Check sheet for the modelled part. Datum: model origin and axes. Units: mm. A direction names the side the tool comes from. Round coordinates to 2 decimals unless told otherwise and drop trailing zeros. Order: outer loops, then holes, each group sorted by start corner. A loop starts at its lowest first (then second) coordinate and runs counter-clockwise, first axis right, second up.
```python
from build123d import *

# Parameters (mm, degrees)
SKETCH_W     = 34
SKETCH_H     = 20
PAD_DEPTH    = 15
SKETCH001_R  = 0.8
PAD001_DEPTH = 2
FILLET_R     = 1
FILLET001_R  = 0.5


with BuildPart() as part:
    # Sketch → Pad (new body)
    with BuildSketch(Plane.XZ):
        with Locations((18.71189, -10.724301)):
            Rectangle(SKETCH_W, SKETCH_H)
    extrude(amount=PAD_DEPTH)

    # Sketch001 → Pad001 (join)
    with BuildSketch(Plane.XZ):
        with Locations((4.01189, -13.224301)):
            Circle(SKETCH001_R)
        with Locations((4.01189, -8.224301)):
            Circle(SKETCH001_R)
        with Locations((33.41189, -18.424301)):
            Circle(SKETCH001_R)
        with Locations((33.41189, -3.024301)):
            Circle(SKETCH001_R)
    extrude(amount=-PAD001_DEPTH)

    # Fillet
    fillet_edges = [part.edges().sort_by_distance(p)[0] for p in [
        (35.71189, -7.5, -20.724301),
        (18.71189, -15, -20.724301),
        (1.71189, -7.5, -20.724301),
        (18.71189, 0, -20.724301),
        (35.71189, -15, -10.724301),
        (35.71189, 0, -10.724301),
        (18.71189, -15, -0.724301),
        (35.71189, -7.5, -0.724301),
        (1.71189, -7.5, -0.724301),
        (1.71189, -15, -10.724301),
        (1.71189, 0, -10.724301),
        (18.71189, 0, -0.724301),
    ]]
    fillet(fillet_edges, radius=FILLET_R)

    # Fillet001
    fillet001_edges = [part.edges().sort_by_distance(p)[0] for p in [
        (3.21189, 2, -13.224301),
        (3.21189, 2, -8.224301),
        (32.61189, 2, -3.024301),
        (32.61189, 2, -18.424301),
    ]]
    fillet(fillet001_edges, radius=FILLET001_R)


solid = part.part
```
Item 1: Sectioned sample at A-A (z = -16.75). Record the cut outline in (x, y).
Answer:
outline: (1.71, -14) arc R1 ccw to (2.71, -15) - (34.71, -15) arc R1 ccw to (35.71, -14) - (35.71, -1) arc R1 ccw to (34.71, 0) - (2.71, 0) arc R1 ccw to (1.71, -1) - close
Item 2: Scan line: line 1 along Y through (x, z) = (28, -9.75). Record every from-to range of solid material in increasing order.
Answer:
line 1: y = -15 to 0
Item 3: Go/stop test with a flat-tipped pin: P1, Ø10, axis at x = 18.5, z = -12, coming from the +Y side. Record where the tip stops, or that it passes through.
Answer:
P1: stops at y = 0
Item 4: Sectioned sample at B-B (x = 13). Record the cut outline in (y, z).
Answer:
outline: (-15, -19.72) arc R1 ccw to (-14, -20.72) - (-1, -20.72) arc R1 ccw to (0, -19.72) - (0, -1.72) arc R1 ccw to (-1, -0.72) - (-14, -0.72) arc R1 ccw to (-15, -1.72) - close
Item 5: Access from +Z, -Z, +X, -X, +Y, -Y to the whole of each face (thin tool, end or side, straight path). Record for faces 5 (the cylindrical face through (18.94, -14.7, -20.44)), 6 (the flat face through (18, 0, -11)).
Answer:
face 5: -Z, +X, -X, -Y
face 6: +Y
Item 6: Release check for a two-part mould opening along Z. For faces 1 (the cylindrical face through (1.997, -7.591, -1.025)), 2 (the flat face through (18, -7, -20.724)), 3 (the flat face through (1.712, -7, -11)), 4 (the cylindrical face through (3.422, 0.74, -7.684)) record: released by +Z, released by -Z, zero draft, split by the parting line, or undercut.
Answer:
face 1: released by +Z
face 2: released by -Z
face 3: zero draft
face 4: undercut
